CAD build for the part. Positions are in the model's coordinates, mm. A direction names the side the tool comes from. Coordinates: 2 decimals unless noted, no trailing zeros. Write each loop counter-clockwise with the first axis right and the second up, starting at its lowest first coordinate (ties: lowest second). Pieces come first, ordered by that corner, then holes. Notation, with made-up numbers: M 60.25,63 L 106.25,63 A28 ccw 106.25,81 Z; hole C 5.5,30.25 d7. An arc over 180 degrees is marked long. Put each result on its own line as item: value. Start each with the question number.
```python
from build123d import *

# Parameters (mm, degrees)
EXTRUDE_2_DEPTH     = 1
SKETCH_2_R          = 2.5
EXTRUDE_3_DEPTH     = 2
SKETCH_3_R          = 1.5
CUT_EXTRUDE_1_DEPTH = 2
SKETCH_4_R          = 0.75
CUT_EXTRUDE_2_DEPTH = 2
CUT_EXTRUDE_START   = 2.5
SKETCH_5_R          = 1.5
CUT_EXTRUDE_3_DEPTH = 2
SKETCH_6_R          = 0.5
SKETCH_6_R_2        = 0.506721332
CUT_EXTRUDE_6_DEPTH = 2


with BuildPart() as part:
    # 草图1 → 凸台-拉伸2 (new body)
    with BuildSketch(Plane(origin=(0, 0, 0), x_dir=(1, 0, 0), z_dir=(0, 1, 0))):
        with BuildLine():
            ThreePointArc((-13, 1.5), (-14.5, 0), (-13, -1.5))
            Line((-13, -1.5), (0, -2.5))
            Line((0, -2.5), (13, -1.5))
            ThreePointArc((13, -1.5), (14.5, 0), (13, 1.5))
            Line((13, 1.5), (0, 2.5))
            Line((0, 2.5), (-13, 1.5))
        make_face()
    extrude(amount=EXTRUDE_2_DEPTH)

    # 草图2 → 凸台-拉伸3 (add)
    with BuildSketch(Plane(origin=(0, 0, 0), x_dir=(1, 0, 0), z_dir=(0, 1, 0))):
        with Locations(Location((0, 0, 0), (0, 0, 270))):
            Circle(SKETCH_2_R)
    extrude(amount=-EXTRUDE_3_DEPTH)

    # 草图3 → 切除-拉伸1 (cut)
    with BuildSketch(Plane(origin=(0, 0, 0), x_dir=(1, 0, 0), z_dir=(0, 1, 0))):
        with Locations(Location((0, 0, 0), (0, 0, 270))):
            Circle(SKETCH_3_R)
    extrude(amount=-CUT_EXTRUDE_1_DEPTH, mode=Mode.SUBTRACT)

    # 草图4 → 切除-拉伸2 (cut)
    with BuildSketch(Plane(origin=(0, 0, 0), x_dir=(1, 0, 0), z_dir=(0, 1, 0))):
        with Locations(Location((0, 0, 0), (0, 0, 270))):
            Circle(SKETCH_4_R)
    extrude(amount=CUT_EXTRUDE_2_DEPTH, mode=Mode.SUBTRACT)

    # 草图5 → 切除-拉伸3 (cut)
    with BuildSketch(Plane(origin=(0, 0, 0), x_dir=(1, 0, 0), z_dir=(0, 1, 0)).offset(CUT_EXTRUDE_START)):
        with Locations(Location((0, 0, 0), (0, 0, 270))):
            Circle(SKETCH_5_R)
    extrude(amount=-CUT_EXTRUDE_3_DEPTH, mode=Mode.SUBTRACT)

    # 草图6 → 切除-拉伸6 (cut)
    with BuildSketch(Plane(origin=(0, 0, 0), x_dir=(1, 0, 0), z_dir=(0, 1, 0))):
        with Locations(Location((13, 0, 0), (0, 0, 270))):
            Circle(SKETCH_6_R)
        with Locations(Location((-13, 0, 0), (0, 0, 270))):
            Circle(SKETCH_6_R)
        with Locations(Location((11, 0, 0), (0, 0, 270))):
            Circle(SKETCH_6_R)
        with Locations(Location((9, 0, 0), (0, 0, 270))):
            Circle(SKETCH_6_R)
        with Locations(Location((-11, 0, 0), (0, 0, 270))):
            Circle(SKETCH_6_R)
        with Locations(Location((-9, 0, 0), (0, 0, 270))):
            Circle(SKETCH_6_R_2)
    extrude(amount=CUT_EXTRUDE_6_DEPTH, mode=Mode.SUBTRACT)


solid = part.part
```
(1) Slice it at D-D, the plane x = -9. Write the cut outline in (y, z), then the cut area to 3 significant figures.
(2) Slice it at B-B, the plane y = -1.5. Write the cut outline in (x, z), then the cut area to 3 significant figures.
(3) Drill centre lines: line 1 (Z direction, x = -13, y = 0.3); line 2 (X direction, y = -0.65, z = 0); line 3 (Y direction, x = -7, z = -1.5). Where is each one in solid material? Low to high. Write a range as [from, to].
(4) Drop flat-ended pins along their axis: pin 1 (2.5 mm diameter, centred on x = 0, z = 0, fed in from +Y); pin 2 (3 mm diameter, centred on x = -4, z = 0.5, fed in from -Y). Give the stop position or say it passes through.
(5) Which spindle directions (+Z, -Z, +X, -X, +Y, -Y) get a long thin tool onto all of the face, cutting with end or side? Do faces 5 (the face through (0.45, -0.99, 1.43)), 6 (the face through (1, 0.5, 0)), 7 (the face through (0.225, 0.246, 0.715)). Say none if no direction does.
(6) Slice it at C-C, the plane z = 1. Write the cut outline in (x, y), then the cut area to 3 significant figures.
(7) Two-plate mould, pull along X, no slides. Class faces 1 (the face through (0, 1, 2)), 2 (the face through (-11.488, 0.493, -0.108)), 3 (the face through (-2.44, -0.99, -0.54)), 4 (the face through (6.409, 0.493, 2.007)): +X half, -X half, draft (parallel to the pull), parting line (faces both ways), or undercut.
(8) Slice it at A-A, the plane x = 9. Write the cut outline in (y, z).
Result set:
1. outline: M 0,-1.81 L 1,-1.81 L 1,-0.51 L 0,-0.51 Z; M 0,0.51 L 1,0.51 L 1,1.81 L 0,1.81 Z
1. area: 2.60 mm^2
2. outline: C 0,0 d5; hole C 0,0 d3
2. area: 12.6 mm^2
3. line 1: z = [-1.5, -0.5], [0.5, 1.5]
3. line 2: x = [-2.5, -1.5], [1.5, 2.5]
3. line 3: y = [0, 1]
4. pin 1: stops at y = 0.5
4. pin 2: stops at y = 0
5. face 5: -Y
5. face 6: +Y
5. face 7: +Y, -Y
6. outline: M -14.12,0 L -2.29,0 L -2.29,-2 L -1.12,-2 L -1.12,0 L 1.12,0 L 1.12,-2 L 2.29,-2 L 2.29,0 L 14.12,0 L 14.12,1 L 1.12,1 L 1.12,0.5 L -1.12,0.5 L -1.12,1 L -14.12,1 Z
6. area: 31.8 mm^2
7. face 1: draft
7. face 2: undercut
7. face 3: parting line
7. face 4: +X half
8. outline: M 0,-1.81 L 1,-1.81 L 1,-0.5 L 0,-0.5 Z; M 0,0.5 L 1,0.5 L 1,1.81 L 0,1.81 Z
